Read the model definition and answer for the solid it produces. Units are mm, in the model's axes. A direction names the side the tool comes from. Coordinates: 2 decimals unless noted, no trailing zeros. Write each loop counter-clockwise with the first axis right and the second up, starting at its lowest first coordinate (ties: lowest second). Pieces come first, ordered by that corner, then holes.
(1) Find the intervals of material crossed by probe 1 along Y at (x, z) = (18, -58); probe 2 along X at (y, z) = (5.5, -11); probe 3 along X at (y, z) = (11.75, -49), in increasing order.
(2) Section A-A on y = 10.25 is taken. Write down the section's boundary in (x, z).
(3) The mould has two halves that part along Z. Classify faces 1 (the flat face through (0, 17, 94)), 2 (the flat face through (20, 27.5, 1)), 3 (the flat face through (-20, 18, 80)): +Z half, -Z half, draft (parallel to the pull), parting line (faces both ways), or undercut.
(4) Section B-B on x = -4.5 is taken. Write down the section's boundary in (y, z), then the cut area to 3 significant figures.
(5) Which of the six approach directions +Z, -Z, +X, -X, +Y, -Y give full straight-line access (tool end or side, diameter ignored) to faces 4 (the flat face through (0, 17, -94)), 5 (the flat face through (20, 2, 1)), 6 (the flat face through (0, 17, -97))?
(6) Given pin 1 (2.5 mm diameter, centred on y = 3, z = -39, fed in from -X); pin 2 (0.9 mm diameter, centred on x = 21, z = -28.5, fed in from +Y); pin 3 (4 mm diameter, centred on x = 11.5, y = 8.5, fed in from -Z), each flat-ended and moving along its own axis, determine where each tip first touches the part or whether it passes through.
Autodesk Inventor part; units mm, degrees
ref_plane "YZ Plane" through (0, 0, 0) normal (1, 0, 0) x (0, 1, 0)
ref_plane "XZ Plane" through (0, 0, 0) normal (0, 1, 0) x (-1, 0, 0)
ref_plane "XY Plane" through (0, 0, 0) normal (0, 0, 1) x (1, 0, 0)
sketch "Sketch2" plane through (0, 0, 0) normal (0, 1, 0) x (-1, 0, 0)
  line L0 (-20, -100) -> (20, -100)
  line L1 (20, -100) -> (20, 100)
  line L2 (20, 100) -> (-20, 100)
  line L3 (-20, 100) -> (-20, -100)
  line L4 (-20, -100) -> (20, 100) construction
  line L5 (20, -100) -> (-20, 100) construction
  point P0 (0, 0)
  dimension "d0" = 40
  dimension "d1" = 200
extrude "Extrusion1" add sketch "Sketch2" along normal blind 5
sketch "Sketch3" plane through (0, 5, 0) normal (0, 1, 0) x (1, 0, 0)
  line L0 (17, 97) -> (-17, 97)
  line L1 (-17, 97) -> (-17, -97)
  line L2 (-17, -97) -> (17, -97)
  line L3 (17, -97) -> (17, 97)
  line L4 (17, 97) -> (-17, -97) construction
  line L5 (-17, 97) -> (17, -97) construction
  line L6 (-20, 100) -> (-20, -100)
  line L7 (-20, -100) -> (20, -100)
  line L8 (14, 94) -> (-14, 94)
  line L9 (-14, 94) -> (-14, -94)
  line L10 (-14, -94) -> (14, -94)
  line L11 (14, -94) -> (14, 94)
  line L12 (14, 94) -> (-14, -94) construction
  line L13 (-14, 94) -> (14, -94) construction
  point P0 (0, 0)
  dimension "d4" = 3
  dimension "d5" = 3
  dimension "d6" = 3
  dimension "d7" = 3
extrude "Extrusion2" add sketch "Sketch3" along normal blind 25
fillet "Fillet1" radius 2 8 edges at (17, 17.5, 97) (-17, 17.5, 97) (-20, 2.5, 100) (20, 2.5, 100) (17, 17.5, -97) (-17, 17.5, -97) (20, 2.5, -100) (-20, 2.5, -100)
sketch "Sketch4" plane through (17, 5, 95) normal (1, 0, 0) x (0, 0, -1)
  line L0 (5, 22.5) -> (185, 22.5)
  line L1 (185, 22.5) -> (185, 2.5)
  line L2 (185, 2.5) -> (5, 2.5)
  line L3 (5, 2.5) -> (5, 22.5)
  line L4 (190, 25) -> (190, 0)
  line L5 (0, 25) -> (190, 25)
  line L6 (0, 0) -> (0, 25)
  line L7 (190, 0) -> (0, 0)
  line L8 (-5, 0) -> (-5, -5)
  line L9 (195, -5) -> (195, 0)
  point P0 (95, -5)
  point P1 (0, 12.5)
  dimension "d42" = 10
  dimension "d43" = 10
  dimension "d44" = 20
  dimension "d45" = 10
extrude "Extrusion3" add sketch "Sketch4" along normal blind 6 contours L0 L1 L2 L3
sketch "Sketch5" plane through (17, 7.5, -90) normal (0, 0, -1) x (-1, 0, 0)
  line L0 (0, 20) -> (0, 0)
  line L1 (0, 20) -> (-6, 20)
  line L2 (-6, 0) -> (-6, 20)
  line L3 (0, 0) -> (-6, 0)
  line L4 (-6, 12.5) -> (-3, 12.5)
  line L5 (-3, 12.5) -> (-3, 7.5)
  line L6 (-3, 7.5) -> (-6, 7.5)
  line L7 (-6, 7.5) -> (-6, 12.5)
  line L8 (0, 15) -> (-3, 15)
  line L9 (-3, 15) -> (-3, 5)
  line L10 (-3, 5) -> (0, 5)
  line L11 (0, 5) -> (0, 15)
  point P0 (17, -7.5)
  point P1 (-4.5, 7.5)
  point P2 (-4.5, 12.5)
  point P3 (-6, 7.5)
  point P4 (-3, 7.5)
  point P5 (0, 5)
  point P6 (-1.5, 15)
  dimension "d17" = 3
  dimension "d20" = 5
  dimension "d21" = 5
  dimension "d46" = 2.5
  dimension "d47" = 2.5
extrude "Extrusion4" cut sketch "Sketch5" against normal blind 170 contours L0 L10 L9 L5 L8 | L4 L5 L6 L2
sketch "Sketch6" plane through (-17, 5, -95) normal (-1, 0, 0) x (0, 0, 1)
  line L0 (0, 0) -> (0, 25)
  line L1 (190, 0) -> (0, 0)
  line L2 (190, 25) -> (190, 0)
  line L3 (0, 25) -> (190, 25)
  line L4 (5, 17.5) -> (175, 17.5)
  line L5 (175, 17.5) -> (175, 7.5)
  line L6 (175, 7.5) -> (5, 7.5)
  line L7 (5, 7.5) -> (5, 17.5)
  line L8 (195, -5) -> (195, 0)
  line L9 (-5, 0) -> (-5, -5)
  point P0 (95, -5)
  point P1 (0, 12.5)
  dimension "d48" = 20
  dimension "d49" = 10
  dimension "d50" = 5
  dimension "d51" = 10
extrude "Extrusion5" add sketch "Sketch6" along normal blind 6 contours L4 L5 L6 L7
sketch "Sketch7" plane through (-17, 12.5, 80) normal (0, 0, 1) x (1, 0, 0)
  line L0 (0, 10) -> (0, 0)
  line L1 (0, 10) -> (-6, 10)
  line L2 (-6, 0) -> (-6, 10)
  line L3 (0, 0) -> (-6, 0)
  line L4 (0, 10) -> (-3, 10)
  line L5 (-3, 10) -> (-3, 7.5)
  line L6 (-3, 7.5) -> (0, 7.5)
  line L7 (0, 7.5) -> (0, 10)
  line L8 (0, 0) -> (-3, 0)
  line L9 (-3, 0) -> (-3, 2.5)
  line L10 (-3, 2.5) -> (0, 2.5)
  line L11 (0, 2.5) -> (0, 0)
  point P0 (17, -12.5)
  dimension "d30" = 3
  dimension "d31" = 2.5
  dimension "d32" = 3
  dimension "d33" = 2.5
extrude "Extrusion6" cut sketch "Sketch7" against normal up to surface (170 mm away) contours L0 L6 L5 L1 | L0 L3 L9 L10
fillet "Fillet3" radius 1 4 edges at (-18.5, 20, -90) (-18.5, 15, -90) (-18.5, 20, 80) (-18.5, 15, 80)
fillet "Fillet4" radius 1 4 edges at (-23, 22.5, -5) (-20, 22.5, -5) (-23, 12.5, -5) (-20, 12.5, -5)
fillet "Fillet5" radius 2 3 edges at (23, 17.5, 90) (23, 23.75, -90) (23, 11.25, -90)
fillet "Fillet6" radius 1 9 edges at (-22.7071, 22.2071, 80) (-21.5, 22.5, 80) (-20.2929, 22.2071, 80) (-20, 20.75, 80) (-22.7071, 12.7929, 80) (-21.5, 12.5, 80) (-20.2929, 12.7929, 80) (-20, 14.25, 80) (-23, 17.5, 80)
fillet "Fillet7" radius 1 9 edges at (-20.2929, 22.2071, -90) (-21.5, 22.5, -90) (-22.7071, 22.2071, -90) (-23, 17.5, -90) (-22.7071, 12.7929, -90) (-21.5, 12.5, -90) (-20.2929, 12.7929, -90) (-20, 14.25, -90) (-20, 20.75, -90)
properties part number "module_switch"
Response:
1. probe 1: y = 0 to 5, 7.5 to 12.5, 22.5 to 27.5
1. probe 2: x = -17 to -14, 14 to 17
1. probe 3: x = -17 to -14, 14 to 23
2. outline: (-17, -95) arc R2 ccw to (-15, -97) - (15, -97) arc R2 ccw to (17, -95) - (17, -90) - (21, -90) arc R2 ccw to (23, -88) - (23, 88) arc R2 ccw to (21, 90) - (17, 90) - (17, 95) arc R2 ccw to (15, 97) - (-15, 97) arc R2 ccw to (-17, 95) - close; hole (-14, -94) - (14, -94) - (14, 94) - (-14, 94) - close
3. face 1: undercut
3. face 2: draft
3. face 3: +Z half
4. outline: (0, -100) - (5, -100) - (5, -97) - (30, -97) - (30, -94) - (5, -94) - (5, 94) - (30, 94) - (30, 97) - (5, 97) - (5, 100) - (0, 100) - close
4. area: 1,150 mm2
5. face 4: +Y
5. face 5: +Z, -Z, +X, -Y
5. face 6: -Z, +X, -X, +Y
6. pin 1: stops at x = -20
6. pin 2: stops at y = 27.5
6. pin 3: stops at z = -97
